from build123d import *

# Parameters (mm, degrees)
SKETCH1_W           = 24
SKETCH1_H           = 24
BOSS_EXTRUDE1_DEPTH = 2
SKETCH2_W           = 22
SKETCH2_H           = 22
SKETCH2_W_2         = 20
SKETCH2_H_2         = 20
BOSS_EXTRUDE2_DEPTH = 1
FILLET1_R           = 1
FILLET2_R           = 1
FILLET3_R           = 0.5


with BuildPart() as part:
    # Sketch1 → Boss-Extrude1 (new body)
    with BuildSketch(Plane.XY):
        Rectangle(SKETCH1_W, SKETCH1_H)
    extrude(amount=BOSS_EXTRUDE1_DEPTH)

    # Sketch2 → Boss-Extrude2 (add)
    with BuildSketch(Plane(origin=(0, 0, 0), x_dir=(-1, 0, 0), z_dir=(0, 0, -1))):
        Rectangle(SKETCH2_W, SKETCH2_H)
        Rectangle(SKETCH2_W_2, SKETCH2_H_2, mode=Mode.SUBTRACT)
    extrude(amount=BOSS_EXTRUDE2_DEPTH)

    # Fillet1
    fillet1_edges = [part.edges().sort_by_distance(p)[0] for p in [
        (-12, 0, 2),
        (0, -12, 2),
        (12, 0, 2),
        (0, 12, 2),
    ]]
    fillet(fillet1_edges, radius=FILLET1_R)

    # Fillet2
    # the kernel refuses this fillet: 1 mm, written as the material it takes off along each edge
    with BuildSketch(Plane(origin=(-11, -11, 1), x_dir=(-1, 0, 0), z_dir=(0, -1, 0))) as fillet2_piece_1_section:
        Polygon((0, 0), (FILLET2_R, 0), (FILLET2_R, -FILLET2_R), (0, -FILLET2_R), align=None)
    fillet2_piece_1 = extrude(amount=FILLET2_R, mode=Mode.PRIVATE)
    fillet2_piece_1 = fillet2_piece_1 - Plane(origin=(-11, -11, 1), x_dir=(0.7071067811865475, 0, -0.7071067811865475), z_dir=(0, -1, 0)) * Sphere(FILLET2_R, mode=Mode.PRIVATE)
    add(fillet2_piece_1, mode=Mode.SUBTRACT)
    with BuildSketch(Plane(origin=(-11, 11, 1), x_dir=(0, 1, 0), z_dir=(-1, 0, 0))) as fillet2_piece_2_section:
        Polygon((0, 0), (FILLET2_R, 0), (FILLET2_R, -FILLET2_R), (0, -FILLET2_R), align=None)
    fillet2_piece_2 = extrude(amount=FILLET2_R, mode=Mode.PRIVATE)
    fillet2_piece_2 = fillet2_piece_2 - Plane(origin=(-11, 11, 1), x_dir=(0, -0.7071067811865475, -0.7071067811865475), z_dir=(-1, 0, 0)) * Sphere(FILLET2_R, mode=Mode.PRIVATE)
    add(fillet2_piece_2, mode=Mode.SUBTRACT)
    with BuildSketch(Plane(origin=(11, -11, 1), x_dir=(1, 0, 0), z_dir=(0, -1, 0))) as fillet2_piece_3_section:
        Polygon((0, 0), (FILLET2_R, 0), (FILLET2_R, FILLET2_R), (0, FILLET2_R), align=None)
    fillet2_piece_3 = extrude(amount=FILLET2_R, mode=Mode.PRIVATE)
    fillet2_piece_3 = fillet2_piece_3 - Plane(origin=(11, -11, 1), x_dir=(-0.7071067811865475, 0, -0.7071067811865475), z_dir=(0, -1, 0)) * Sphere(FILLET2_R, mode=Mode.PRIVATE)
    add(fillet2_piece_3, mode=Mode.SUBTRACT)
    with BuildSketch(Plane(origin=(11, 11, 1), x_dir=(0, 1, 0), z_dir=(1, 0, 0))) as fillet2_piece_4_section:
        Polygon((0, 0), (FILLET2_R, 0), (FILLET2_R, FILLET2_R), (0, FILLET2_R), align=None)
    fillet2_piece_4 = extrude(amount=FILLET2_R, mode=Mode.PRIVATE)
    fillet2_piece_4 = fillet2_piece_4 - Plane(origin=(11, 11, 1), x_dir=(0, -0.7071067811865475, -0.7071067811865475), z_dir=(1, 0, 0)) * Sphere(FILLET2_R, mode=Mode.PRIVATE)
    add(fillet2_piece_4, mode=Mode.SUBTRACT)
    with BuildSketch(Plane(origin=(12, 12, -2.5), x_dir=(0, -1, 0), z_dir=(0, 0, 1)), Plane(origin=(12, -12, -2.5), x_dir=(-1, 0, 0), z_dir=(0, 0, 1))) as fillet2_piece_5:
        with BuildLine():
            CenterArc((FILLET2_R, -FILLET2_R), FILLET2_R, 90, 90)
            Line((0, -FILLET2_R), (0, 0))
            Line((0, 0), (FILLET2_R, 0))
        make_face()
    extrude(amount=3.5, mode=Mode.SUBTRACT)
    with BuildSketch(Plane(origin=(-12, -12, -2.5), x_dir=(1, 0, 0), z_dir=(0, 0, 1)), Plane(origin=(-12, 12, -2.5), x_dir=(0, -1, 0), z_dir=(0, 0, 1))) as fillet2_piece_6:
        with BuildLine():
            CenterArc((FILLET2_R, FILLET2_R), FILLET2_R, 180, 90)
            Line((0, FILLET2_R), (0, 0))
            Line((0, 0), (FILLET2_R, 0))
        make_face()
    extrude(amount=3.5, mode=Mode.SUBTRACT)

    # Fillet3
    fillet3_edges = [part.edges().sort_by_distance(p)[0] for p in [
        (-11, -11, -0.5),
        (-11, 11, -0.5),
        (11, 11, -0.5),
        (11, -11, -0.5),
    ]]
    fillet(fillet3_edges, radius=FILLET3_R)


solid = part.part
Check sheet for the modelled part. Datum: model origin and axes. Units: mm. A direction names the side the tool comes from. Give positions to 0.01 mm unless a question says otherwise; leave off trailing zeros. Loops run counter-clockwise (first coordinate to the right, second up) from the corner with the lowest first, then second, coordinate; pieces in that order, holes last. Notation, with made-up numbers: M 35.25,41 L 40.25,41 A25 ccw 40.25,60 Z; hole C 9,65 d10. An arc over 180 degrees is marked long. Answer as a JSON object with one key per item and string values. Group by question number.
Q1. Go/stop test with flat-tipped pins: P1, Ø0.8, axis at x = 1, z = -0.5, coming from the -Y side; P2, Ø7, axis at x = 1, y = -2, coming from the -Z side; P3, Ø0.5, axis at y = -2, z = -0.5, coming from the -X side. Record where each tip stops, or that it passes through.
Q2. Material ranges on line 1 along Y through (x, z) = (8, -0.1); line 2 along Z through (x, y) = (-9.5, 3.25), recorded low to high. Write a range as [from, to].
Q3. Access from +Z, -Z, +X, -X, +Y, -Y to the whole of each face (thin tool, end or side, straight path). Record for faces 1 (the flat face through (11, -0.1, -0.5)), 2 (the flat face through (10, -0.1, -0.5)), 3 (the flat face through (-11, -0.1, -0.5)), 4 (the cylindrical face through (0.154, 11.715, 1.699)).
Q4. Release check for a two-part mould opening along X. For faces 5 (the flat face through (0.1, 10, -0.5)), 6 (the cylindrical face through (11.699, -11.715, 0.493)), 7 (the flat face through (0, 0, 0)), 8 (the flat face through (0.1, 11, -0.5)) record: released by +X, released by -X, zero draft, split by the parting line, or undercut.
Q5. Cross-section at D-D on z = 1.5. Record the cut outline in (x, y).
Q6. Cross-section at A-A on z = -0.45. Record the cut outline in (x, y).
Q7. Cross-section at B-B on y = -6. Record the cut outline in (x, z), then the cut area to 3 significant figures.
Evaluation:
{
 "1": {"P1": "stops at y = -11", "P2": "stops at z = 0", "P3": "stops at x = -11"},
 "2": {"line 1": "y = [-11, -10], [10, 11]", "line 2": "z = [0, 2]"},
 "3": {"face 1": "-Z, +X, +Y, -Y", "face 2": "-Z", "face 3": "-Z, -X, +Y, -Y", "face 4": "+Z, +X, -X, +Y"},
 "4": {"face 5": "undercut", "face 6": "released by +X", "face 7": "undercut", "face 8": "zero draft"},
 "5": {"outline": "M -11.87,-11 A0.87 ccw -11,-11.87 L 11,-11.87 A0.87 ccw 11.87,-11 L 11.87,11 A0.87 ccw 11,11.87 L -11,11.87 A0.87 ccw -11.87,11 Z"},
 "6": {"outline": "M -11,-10.5 A0.5 ccw -10.5,-11 L 10.5,-11 A0.5 ccw 11,-10.5 L 11,10.5 A0.5 ccw 10.5,11 L -10.5,11 A0.5 ccw -11,10.5 Z; hole M -10,-10 L 10,-10 L 10,10 L -10,10 Z"},
 "7": {"outline": "M -12,0 L -11,0 L -11,-1 L -10,-1 L -10,0 L 10,0 L 10,-1 L 11,-1 L 11,0 L 12,0 L 12,1 A1 ccw 11,2 L -11,2 A1 ccw -12,1 Z", "area": "49.6 mm2"}
}
